```python
from build123d import *

# Parameters (mm, degrees)
BOSS_EXTRUDE1_DEPTH = 12.065
SKETCH2_6_R         = 9.525
SKETCH2_6_R_2       = 7.025
SKETCH2_6_R_3       = 3.4
CUT_EXTRUDE1_DEPTH  = 68.25
SKETCH2_R           = 9.525
SKETCH2_R_2         = 7.025
SKETCH2_R_3         = 3.4
BOSS_EXTRUDE2_DEPTH = 15.25
SKETCH2_8_R         = 7.025
SKETCH2_8_R_2       = 3.4
BOSS_EXTRUDE3_DEPTH = 7.25


with BuildPart() as part:
    # Sketch1 → Boss-Extrude1 (new, symmetric)
    with BuildSketch(Plane(origin=(0, 0, 0), x_dir=(0, 0, -1), z_dir=(1, 0, 0))):
        with BuildLine():
            Line((38.1, 0), (50.8, 0))
            ThreePointArc((50.8, 0), (0, 50.8), (-50.8, 0))
            Line((-50.8, 0), (-38.1, 0))
            ThreePointArc((-38.1, 0), (0, 38.1), (38.1, 0))
        make_face()
    extrude(amount=BOSS_EXTRUDE1_DEPTH, both=True)

    # Sketch2_6 → Cut-Extrude1 (cut)
    # profile 1 of 15: a face of its own
    with BuildSketch(Plane.XZ):
        with BuildLine():
            Line((9.525, -50.8), (7.025, -50.8))
            ThreePointArc((7.025, -50.8), (0, -57.825), (-7.025, -50.8))
            Line((-7.025, -50.8), (-9.525, -50.8))
            ThreePointArc((-9.525, -50.8), (0, -60.325), (9.525, -50.8))
        make_face()
    # profile 2 of 15: a face of its own
    with BuildSketch(Plane.XZ):
        with BuildLine():
            ThreePointArc((-7.025, -50.8), (0, -43.775), (7.025, -50.8))
            Line((7.025, -50.8), (9.525, -50.8))
            ThreePointArc((9.525, -50.8), (0, -41.275), (-9.525, -50.8))
            Line((-9.525, -50.8), (-7.025, -50.8))
        make_face()
    # profile 3 of 15: a face of its own
    with BuildSketch(Plane.XZ):
        with BuildLine():
            Line((9.525, -50.8), (7.025, -50.8))
            ThreePointArc((7.025, -50.8), (0, -57.825), (-7.025, -50.8))
            Line((-7.025, -50.8), (-9.525, -50.8))
            ThreePointArc((-9.525, -50.8), (0, -60.325), (9.525, -50.8))
        make_face()
    # profile 4 of 15: a face of its own
    with BuildSketch(Plane.XZ):
        with BuildLine():
            ThreePointArc((-7.025, -50.8), (0, -43.775), (7.025, -50.8))
            Line((7.025, -50.8), (9.525, -50.8))
            ThreePointArc((9.525, -50.8), (0, -41.275), (-9.525, -50.8))
            Line((-9.525, -50.8), (-7.025, -50.8))
        make_face()
    # profile 5 of 15: a face of its own
    with BuildSketch(Plane.XZ):
        with BuildLine():
            Line((7.025, -50.8), (3.4, -50.8))
            ThreePointArc((3.4, -50.8), (0, -54.2), (-3.4, -50.8))
            Line((-3.4, -50.8), (-7.025, -50.8))
            ThreePointArc((-7.025, -50.8), (0, -57.825), (7.025, -50.8))
        make_face()
    # profile 6 of 15: a face of its own
    with BuildSketch(Plane.XZ):
        with BuildLine():
            ThreePointArc((-3.4, -50.8), (0, -47.4), (3.4, -50.8))
            Line((3.4, -50.8), (7.025, -50.8))
            ThreePointArc((7.025, -50.8), (0, -43.775), (-7.025, -50.8))
            Line((-7.025, -50.8), (-3.4, -50.8))
        make_face()
    # profile 7 of 15: a face of its own
    with BuildSketch(Plane.XZ):
        with BuildLine():
            Line((7.025, -50.8), (3.4, -50.8))
            ThreePointArc((3.4, -50.8), (0, -54.2), (-3.4, -50.8))
            Line((-3.4, -50.8), (-7.025, -50.8))
            ThreePointArc((-7.025, -50.8), (0, -57.825), (7.025, -50.8))
        make_face()
    # profile 8 of 15: a face of its own
    with BuildSketch(Plane.XZ):
        with BuildLine():
            ThreePointArc((-3.4, -50.8), (0, -47.4), (3.4, -50.8))
            Line((3.4, -50.8), (7.025, -50.8))
            ThreePointArc((7.025, -50.8), (0, -43.775), (-7.025, -50.8))
            Line((-7.025, -50.8), (-3.4, -50.8))
        make_face()
    # profile 9 of 15: a face of its own
    with BuildSketch(Plane.XZ):
        with BuildLine():
            Line((-3.4, -50.8), (3.4, -50.8))
            ThreePointArc((3.4, -50.8), (0, -47.4), (-3.4, -50.8))
        make_face()
    # profile 10 of 15: a face of its own
    with BuildSketch(Plane.XZ):
        with BuildLine():
            ThreePointArc((-3.4, -50.8), (0, -54.2), (3.4, -50.8))
            Line((3.4, -50.8), (-3.4, -50.8))
        make_face()
    # profile 11 of 15: a face of its own
    with BuildSketch(Plane.XZ):
        with BuildLine():
            Line((-3.4, -50.8), (3.4, -50.8))
            ThreePointArc((3.4, -50.8), (0, -47.4), (-3.4, -50.8))
        make_face()
    # profile 12 of 15: a face of its own
    with BuildSketch(Plane.XZ):
        with BuildLine():
            ThreePointArc((-3.4, -50.8), (0, -54.2), (3.4, -50.8))
            Line((3.4, -50.8), (-3.4, -50.8))
        make_face()
    # profile 13 of 15: a face of its own
    with BuildSketch(Plane.XZ):
        with Locations((0, 50.8)):
            Circle(SKETCH2_6_R)
        with Locations((0, 50.8)):
            Circle(SKETCH2_6_R_2, mode=Mode.SUBTRACT)
    # profile 14 of 15: a face of its own
    with BuildSketch(Plane.XZ):
        with Locations((0, 50.8)):
            Circle(SKETCH2_6_R_2)
        with Locations((0, 50.8)):
            Circle(SKETCH2_6_R_3, mode=Mode.SUBTRACT)
    # profile 15 of 15: a face of its own
    with BuildSketch(Plane.XZ):
        with Locations((0, 50.8)):
            Circle(SKETCH2_6_R_3)
    extrude(amount=-CUT_EXTRUDE1_DEPTH, mode=Mode.SUBTRACT)

    # Sketch2 → Boss-Extrude2 (add)
    # profile 1 of 7: a face of its own
    with BuildSketch(Plane.XZ):
        with BuildLine():
            Line((9.525, -50.8), (7.025, -50.8))
            ThreePointArc((7.025, -50.8), (0, -57.825), (-7.025, -50.8))
            Line((-7.025, -50.8), (-9.525, -50.8))
            ThreePointArc((-9.525, -50.8), (0, -60.325), (9.525, -50.8))
        make_face()
    # profile 2 of 7: a face of its own
    with BuildSketch(Plane.XZ):
        with BuildLine():
            ThreePointArc((-7.025, -50.8), (0, -43.775), (7.025, -50.8))
            Line((7.025, -50.8), (9.525, -50.8))
            ThreePointArc((9.525, -50.8), (0, -41.275), (-9.525, -50.8))
            Line((-9.525, -50.8), (-7.025, -50.8))
        make_face()
    # profile 3 of 7: a face of its own
    with BuildSketch(Plane.XZ):
        with BuildLine():
            Line((9.525, -50.8), (7.025, -50.8))
            ThreePointArc((7.025, -50.8), (0, -57.825), (-7.025, -50.8))
            Line((-7.025, -50.8), (-9.525, -50.8))
            ThreePointArc((-9.525, -50.8), (0, -60.325), (9.525, -50.8))
        make_face()
    # profile 4 of 7: a face of its own
    with BuildSketch(Plane.XZ):
        with BuildLine():
            ThreePointArc((-7.025, -50.8), (0, -43.775), (7.025, -50.8))
            Line((7.025, -50.8), (9.525, -50.8))
            ThreePointArc((9.525, -50.8), (0, -41.275), (-9.525, -50.8))
            Line((-9.525, -50.8), (-7.025, -50.8))
        make_face()
    # profile 5 of 7: a face of its own
    with BuildSketch(Plane.XZ):
        with Locations((0, 50.8)):
            Circle(SKETCH2_R)
        with Locations(Location((0, 50.8, 0), (0, 0, 270))):
            Circle(SKETCH2_R_2, mode=Mode.SUBTRACT)
    # profile 6 of 7: a face of its own
    with BuildSketch(Plane.XZ):
        with Locations((0, 50.8)):
            Circle(SKETCH2_R_3)
    # profile 7 of 7: a face of its own
    with BuildSketch(Plane.XZ):
        with Locations((0, -50.8)):
            Circle(SKETCH2_R_3)
    extrude(amount=-BOSS_EXTRUDE2_DEPTH)


with BuildPart() as boss_extrude2_kept_piece:
    # of the separate pieces the step leaves, the one the design keeps (boss_extrude2_pieces_kept)
    add(part.part.solids().sort_by_distance((-9.525, 0, -50.8))[0])

    # Sketch2_8 → Boss-Extrude3 (add)
    # profile 1 of 5: a face of its own
    with BuildSketch(Plane.XZ):
        with Locations(Location((0, 50.8, 0), (0, 0, 270))):
            Circle(SKETCH2_8_R)
        with Locations(Location((0, 50.8, 0), (0, 0, 270))):
            Circle(SKETCH2_8_R_2, mode=Mode.SUBTRACT)
    # profile 2 of 5: a face of its own
    with BuildSketch(Plane.XZ):
        with BuildLine():
            Line((7.025, -50.8), (3.4, -50.8))
            ThreePointArc((3.4, -50.8), (0, -54.2), (-3.4, -50.8))
            Line((-3.4, -50.8), (-7.025, -50.8))
            ThreePointArc((-7.025, -50.8), (0, -57.825), (7.025, -50.8))
        make_face()
    # profile 3 of 5: a face of its own
    with BuildSketch(Plane.XZ):
        with BuildLine():
            ThreePointArc((-3.4, -50.8), (0, -47.4), (3.4, -50.8))
            Line((3.4, -50.8), (7.025, -50.8))
            ThreePointArc((7.025, -50.8), (0, -43.775), (-7.025, -50.8))
            Line((-7.025, -50.8), (-3.4, -50.8))
        make_face()
    # profile 4 of 5: a face of its own
    with BuildSketch(Plane.XZ):
        with BuildLine():
            Line((7.025, -50.8), (3.4, -50.8))
            ThreePointArc((3.4, -50.8), (0, -54.2), (-3.4, -50.8))
            Line((-3.4, -50.8), (-7.025, -50.8))
            ThreePointArc((-7.025, -50.8), (0, -57.825), (7.025, -50.8))
        make_face()
    # profile 5 of 5: a face of its own
    with BuildSketch(Plane.XZ):
        with BuildLine():
            ThreePointArc((-3.4, -50.8), (0, -47.4), (3.4, -50.8))
            Line((3.4, -50.8), (7.025, -50.8))
            ThreePointArc((7.025, -50.8), (0, -43.775), (-7.025, -50.8))
            Line((-7.025, -50.8), (-3.4, -50.8))
        make_face()
    extrude(amount=-BOSS_EXTRUDE3_DEPTH)


solid = boss_extrude2_kept_piece.part
```
The listing builds one solid part. Answer for the finished solid, in the listing's coordinates (mm). A direction names the side the tool comes from. Coordinates: 2 decimals unless noted, no trailing zeros. Write each loop counter-clockwise with the first axis right and the second up, starting at its lowest first coordinate (ties: lowest second). Pieces come first, ordered by that corner, then holes. Notation, with made-up numbers: M 77.5,81.25 L 128.5,81.25 A22 cw 128.5,98.25 Z; hole C -23,-22 d5. An arc over 180 degrees is marked long. Use a Markdown table: item, result. Add a question column.
1. Which of the six approach directions +Z, -Z, +X, -X, +Y, -Y give full straight-line access (tool end or side, diameter ignored) to faces 1 (the flat face through (3.2, 7.25, 52.5)), 2 (the flat face through (12.065, 43, 1)), 3 (the flat face through (-1, 15.25, -58))?
2. Straight lines are drawn through the part: line 1 along X through (y, z) = (13.5, -50.8) (3 decimals); line 2 along Z through (x, y) = (-2.75, 9); line 3 along Y through (x, z) = (6, -53). For each, find the intervals that lie inside material, in ascending order. Write a range as [from, to].
3. For a pull along Z with two mould halves and no side action, classify faces 4 (the flat face through (-4, 15.25, 44)), 5 (the cylindrical face through (0.1, 3.6, 54.2)), 6 (the cylindrical face through (2.11, 11.19, 44.1)), 7 (the cylindrical face through (-0.176, 20.736, 41.277)) as +Z half, -Z half, draft (parallel to the pull), parting line (faces both ways), or undercut.
4. Section B-B (y = 6) is taken. Give the vertices of the cut face in (x, z) (3 decimals), plus the area to 3 significant figures.
5. Section C-C (y = 26.5) is taken. Give the vertices of the cut face in (x, z) (3 decimals).
6. Section A-A (x = 0) is taken. Give the vertices of the cut face in (y, z) (3 decimals).
7. Section D-D (z = 45.5) is taken. Give the vertices of the cut face in (x, y) (3 decimals).
8. Given P1, Ø12, axis at x = 8, y = 36.5, coming from the -Z side (3 decimals); P2, Ø5.5, axis at x = -3, z = -49.5, coming from the +Y side; P3, Ø7, axis at x = 3.5, z = 49.5, coming from the +Y side, each flat-ended and moving along its own axis, determine where each tip first touches the part or whether it passes through.
Data:
| question | item | result |
|---|---|---|
| 1 | face 1 | +Y |
| 1 | face 2 | +Z, -Z, +X, +Y, -Y |
| 1 | face 3 | -Z, +Y |
| 2 | line 1 | x = [-9.525, -7.025], [7.025, 9.525] |
| 2 | line 2 | z = [-59.92, -57.26], [-44.34, -37.02], [37.02, 44.34], [57.26, 59.92] |
| 2 | line 3 | y = [0, 7.25] |
| 3 | face 4 | draft |
| 3 | face 5 | undercut |
| 3 | face 6 | undercut |
| 3 | face 7 | +Z half |
| 4 | outline | M -12.065,-50.444 L -9.518,-50.444 A9.525 ccw long 9.518,-50.444 L 12.065,-50.444 L 12.065,-37.625 L -12.065,-37.625 Z; M -12.065,37.625 L 12.065,37.625 L 12.065,50.444 L 9.518,50.444 A9.525 ccw long -9.518,50.444 L -12.065,50.444 Z; hole C 0,-50.8 d6.8; hole C 0,50.8 d6.8 |
| 4 | area | 845 mm2 |
| 5 | outline | M -12.065,-43.34 L -5.923,-43.34 A9.525 cw 5.923,-43.34 L 12.065,-43.34 L 12.065,-27.374 L -12.065,-27.374 Z; M -12.065,27.374 L 12.065,27.374 L 12.065,43.34 L 5.923,43.34 A9.525 cw -5.923,43.34 L -12.065,43.34 Z |
| 6 | outline | M 0,-60.325 L 15.25,-60.325 L 15.25,-57.825 L 7.25,-57.825 L 7.25,-54.2 L 0,-54.2 Z; M 0,-47.4 L 7.25,-47.4 L 7.25,-43.775 L 15.25,-43.775 L 15.25,-41.275 L 29.614,-41.275 A50.8 ccw 29.614,41.275 L 15.25,41.275 L 15.25,43.775 L 7.25,43.775 L 7.25,47.4 L 0,47.4 L 0,38.1 A38.1 cw 0,-38.1 Z; M 0,54.2 L 7.25,54.2 L 7.25,57.825 L 15.25,57.825 L 15.25,60.325 L 0,60.325 Z |
| 7 | outline | M -12.065,0 L 12.065,0 L 12.065,22.592 L 7.914,22.592 L 7.914,15.25 L 4.611,15.25 L 4.611,7.25 L -4.611,7.25 L -4.611,15.25 L -7.914,15.25 L -7.914,22.592 L -12.065,22.592 Z |
| 8 | P1 | stops at z = -40.625 |
| 8 | P2 | stops at y = 7.25 |
| 8 | P3 | stops at y = 15.25 |
